Autodesk Inventor part; units mm, degrees
ref_plane "YZ Plane" through (0, 0, 0) normal (1, 0, 0) x (0, 1, 0)
ref_plane "XZ Plane" through (0, 0, 0) normal (0, 1, 0) x (-1, 0, 0)
ref_plane "XY Plane" through (0, 0, 0) normal (0, 0, 1) x (1, 0, 0)
sketch "Boceto1" plane through (0, 0, 0) normal (0, 1, 0) x (-1, 0, 0)
  arc A0 (19.363, 14.6519) -> (19.2523, 14.77) centre (19.0755, 14.4935) ccw
  arc A1 (19.9736, 14.77) -> (19.863, 14.6519) centre (20.1504, 14.4935) ccw
  ellipse E0 centre (19.613, 24.2247) end of major axis (19.613, 30.2556) minor radius 3.5091 (19.113, 30.1941) -> (18.6267, 18.4369) ccw
  arc A2 (18.6267, 16.2507) -> (19.2422, 15.3368) centre (19.613, 16.2507) ccw
  arc A3 (19.9837, 15.3368) -> (20.5992, 16.2507) centre (19.613, 16.2507) ccw
  line L0 (20.5992, 16.2507) -> (20.5992, 18.4369)
  line L1 (23.3999, 14.52) -> (21.7772, 14.77)
  line L2 (21.7772, 15.27) -> (23.3999, 15.52)
  line L3 (40, 0) -> (0, 0)
  line L4 (18.6267, 16.2507) -> (18.6267, 18.4369)
  ellipse E1 centre (19.613, 24.2247) end of major axis (19.613, 30.2556) minor radius 3.5091 (20.5992, 18.4369) -> (20.113, 30.1941) ccw
  line L5 (21.7772, 14.77) -> (19.9736, 14.77)
  line L6 (19.997, 15.27) -> (21.7772, 15.27)
  line L7 (19.997, 15.27) -> (19.9109, 15.27)
  line L8 (19.9109, 15.27) -> (19.9837, 15.3368)
  line L9 (19.2289, 15.27) -> (19.315, 15.27)
  line L10 (19.315, 15.27) -> (19.2422, 15.3368)
  arc A4 (27.9362, 14.52) -> (27.9362, 15.52) centre (28.4952, 15.02) ccw
  line L11 (23.3999, 15.52) -> (27.9362, 15.52)
  line L12 (23.3999, 14.52) -> (27.9362, 14.52)
  line L13 (15.8494, 15.52) -> (17.4722, 15.27)
  line L14 (17.4722, 14.77) -> (15.8494, 14.52)
  line L15 (17.4722, 15.27) -> (19.2757, 15.27)
  line L16 (19.2523, 14.77) -> (17.4722, 14.77)
  arc A5 (11.3132, 15.52) -> (11.3132, 14.52) centre (10.7541, 15.02) ccw
  line L17 (15.8494, 14.52) -> (11.3132, 14.52)
  line L18 (15.8494, 15.52) -> (11.3132, 15.52)
  line L19 (19.863, 12.8717) -> (20.113, 11.249)
  line L20 (19.113, 11.249) -> (19.363, 12.8717)
  line L21 (20.113, 11.249) -> (20.113, 6.7127)
  arc A6 (19.113, 6.7127) -> (20.113, 6.7127) centre (19.613, 6.1537) ccw
  line L22 (19.113, 11.249) -> (19.113, 6.7127)
  line L23 (19.363, 12.8717) -> (19.363, 14.6519)
  line L24 (19.863, 14.6519) -> (19.863, 12.8717)
  arc A7 (20.113, 33.9983) -> (19.113, 33.9983) centre (19.613, 34.5573) ccw
  line L25 (19.113, 30.1941) -> (19.113, 33.9983)
  line L26 (20.113, 30.1941) -> (20.113, 33.9983)
  line L27 (0, 0) -> (0, 40)
  line L28 (0, 40) -> (40, 40)
  line L29 (40, 40) -> (40, 0)
extrude "Extrusión1" add sketch "Boceto1" along normal blind 5 contours A0 L16 L14 L17 A5 L18 L13 L15 L9 L10 A2 L4 E0 L25 A7 L26 E1 L0 A3 L8 L7 L6 L2 L11 A4 L12 L1 L5 A1 L24 L19 L21 A6 L22 L20 L23 | L3 L27 L28 L29
extrude "Extrusión2" cut sketch "Boceto1" along normal blind 0.2 contours A0 L16 L14 L17 A5 L18 L13 L15 L9 L10 A2 L4 E0 L25 A7 L26 E1 L0 A3 L8 L7 L6 L2 L11 A4 L12 L1 L5 A1 L24 L19 L21 A6 L22 L20 L23
sketch "Boceto2" plane through (0, 0.2, 0) normal (0, -1, 0) x (1, 0, 0)
  arc A0 (-19.113, 33.9983) -> (-20.113, 33.9983) centre (-19.613, 34.5573) ccw
  arc A1 (-11.3132, 14.52) -> (-11.3132, 15.52) centre (-10.7541, 15.02) ccw
  arc A2 (-20.113, 6.7127) -> (-19.113, 6.7127) centre (-19.613, 6.1537) ccw
  arc A3 (-27.9362, 15.52) -> (-27.9362, 14.52) centre (-28.4952, 15.02) ccw
  circle A4 centre (-28.4952, 15.02) radius 0.35
  circle A5 centre (-19.613, 6.1537) radius 0.35
  circle A6 centre (-10.7541, 15.02) radius 0.35
  circle A7 centre (-19.613, 34.5573) radius 0.35
  point P0 (0, 0)
  dimension "d11" = 0.7
  dimension "d12" = 0.7
  dimension "d13" = 0.7
  dimension "d14" = 0.7
extrude "Extrusión3" cut sketch "Boceto2" against normal through all
properties part number "droplet-generator"
Input: part model. Units: mm. Frame: model coordinates. Coordinates: 2 decimals unless noted, no trailing zeros. Answer in a Markdown table with one row per item. Add a question column.
Item 1: Line query: line 1 along X through (y, z) = (0.1, 15.02); line 2 along Y through (x, z) = (-18, 21). Output: solid intervals per line, ascending. Write a range as [from, to].
Item 2: Contact query for a flat-ended pin moving along its axis: P1, Ø4, axis at x = -20.5, z = 26.5, coming from the -Y side. Output: stop coordinate, or through.
Item 3: Mould query, pull axis X, two halves, no side actions, for faces 1 (the flat face through (-40, 2, 20)), 2 (the flat face through (-20, 0.2, 20)), 3 (the flat face through (-24, 0, 20)). Classes: released by +X, released by -X, zero draft, split by the parting line, or undercut.
Recorded:
| question | item | result |
|---|---|---|
| 1 | line 1 | [-40, -29.25], [-10, 0] |
| 1 | line 2 | [0.2, 5] |
| 2 | P1 | y = 0.2 |
| 3 | face 1 | released by -X |
| 3 | face 2 | undercut |
| 3 | face 3 | zero draft |
